Verification items for the finished model (mm, model axes). A direction names the side the tool comes from. Coordinates: 2 decimals unless noted, no trailing zeros. Loops run counter-clockwise (first coordinate to the right, second up) from the corner with the lowest first, then second, coordinate; pieces in that order, holes last. Notation, with made-up numbers: (72.5, 9.25) - (95.5, 9.25) arc R27 ccw to (95.5, 37.25) - close; hole circle Ø6 at (37, 7.25). An arc over 180 degrees is marked (long way). One line per item, written item: value. Start each with the question number.
(1) Section check D-D (z = 265). Record the boundary of the cut face in (x, y).
(2) Section check B-B (z = 12.7). Record the boundary of the cut face in (x, y) (1 decimal).
(3) Draft check along X on faces 1 (the face through (13, 1.587, 155)), 2 (the face through (25.4, 13, 155)), 3 (the face through (0, 13, 155)), 4 (the face through (0.805, 13.463, 198.237)). Enter one of: +X half, -X half, draft (parallel to the pull), parting line (faces both ways), or undercut.
(4) Set-up check for faces 5 (the face through (23.812, 13, 155)), 6 (the face through (0.8, 12.8, 279.4)): record each of +Z, -Z, +X, -X, +Y, -Y from which the full face is reachable in a straight line by a thin tool's end or side.
(5) Section check C-C (x = 10). Record the boundary of the cut face in (y, z).
(6) Section check A-A (z = 88.9). Record the boundary of the cut face in (x, y).
(7) Thickness scan on probe 1 along X at (y, z) = (6.5, 231.5); probe 2 along Y at (x, z) = (1.05, 114.3). Record the ranges inside material, lowest first. Write a range as [from, to].
```python
from build123d import *

# Parameters (mm, degrees)
SKETCH1_W           = 25.4
SKETCH1_H           = 25.4
SKETCH1_W_2         = 22.225
SKETCH1_H_2         = 22.225
BOSS_EXTRUDE1_DEPTH = 314.96
SKETCH3_R           = 2.54
CUT_EXTRUDE2_DEPTH  = 318.00176908
SKETCH4_R           = 2.54
CUT_EXTRUDE3_DEPTH  = 318.00176908


with BuildPart() as part:
    # Sketch1 → Boss-Extrude1 (new body)
    with BuildSketch(Plane.XY):
        with Locations((12.7, 12.7)):
            Rectangle(SKETCH1_W, SKETCH1_H)
        with Locations((12.7, 12.7)):
            Rectangle(SKETCH1_W_2, SKETCH1_H_2, mode=Mode.SUBTRACT)
    extrude(amount=BOSS_EXTRUDE1_DEPTH)

    # Sketch3 → Cut-Extrude2 (cut, through all)
    with BuildSketch(Plane(origin=(0, 25.4, 0), x_dir=(1, 0, 0), z_dir=(0, 1, 0))):
        with Locations(Location((15.875, -302.26, 0), (0, 0, 270))):
            Circle(SKETCH3_R)
        with Locations(Location((15.875, -12.7, 0), (0, 0, 270))):
            Circle(SKETCH3_R)
    extrude(amount=-CUT_EXTRUDE2_DEPTH, mode=Mode.SUBTRACT)

    # Sketch4 → Cut-Extrude3 (cut, through all)
    with BuildSketch(Plane(origin=(25.4, 0, 0), x_dir=(0, 0, -1), z_dir=(1, 0, 0))):
        with Locations((-302.26, 12.7)):
            Circle(SKETCH4_R)
        with Locations((-276.86, 12.7)):
            Circle(SKETCH4_R)
        with Locations((-251.46, 12.7)):
            Circle(SKETCH4_R)
        with Locations((-226.06, 12.7)):
            Circle(SKETCH4_R)
        with Locations((-200.66, 12.7)):
            Circle(SKETCH4_R)
        with Locations(Location((-114.3, 12.7, 0), (0, 0, 180))):
            Circle(SKETCH4_R)
        with Locations(Location((-88.9, 12.7, 0), (0, 0, 180))):
            Circle(SKETCH4_R)
        with Locations(Location((-63.5, 12.7, 0), (0, 0, 180))):
            Circle(SKETCH4_R)
        with Locations(Location((-38.1, 12.7, 0), (0, 0, 180))):
            Circle(SKETCH4_R)
        with Locations(Location((-12.7, 12.7, 0), (0, 0, 180))):
            Circle(SKETCH4_R)
    extrude(amount=-CUT_EXTRUDE3_DEPTH, mode=Mode.SUBTRACT)


solid = part.part
```
Responses:
1. outline: (0, 0) - (25.4, 0) - (25.4, 25.4) - (0, 25.4) - close; hole (1.59, 1.59) - (23.81, 1.59) - (23.81, 23.81) - (1.59, 23.81) - close
2. outline: (0, 0) - (13.3, 0) - (13.3, 1.6) - (1.6, 1.6) - (1.6, 10.2) - (0, 10.2) - close; (0, 15.2) - (1.6, 15.2) - (1.6, 23.8) - (13.3, 23.8) - (13.3, 25.4) - (0, 25.4) - close; (18.4, 0) - (25.4, 0) - (25.4, 10.2) - (23.8, 10.2) - (23.8, 1.6) - (18.4, 1.6) - close; (18.4, 23.8) - (23.8, 23.8) - (23.8, 15.2) - (25.4, 15.2) - (25.4, 25.4) - (18.4, 25.4) - close
3. face 1: undercut
3. face 2: +X half
3. face 3: -X half
3. face 4: draft
4. face 5: +Z, -Z
4. face 6: +X, -X
5. outline: (0, 0) - (1.59, 0) - (1.59, 314.96) - (0, 314.96) - close; (23.81, 0) - (25.4, 0) - (25.4, 314.96) - (23.81, 314.96) - close
6. outline: (0, 0) - (25.4, 0) - (25.4, 10.16) - (23.81, 10.16) - (23.81, 1.59) - (1.59, 1.59) - (1.59, 10.16) - (0, 10.16) - close; (0, 15.24) - (1.59, 15.24) - (1.59, 23.81) - (23.81, 23.81) - (23.81, 15.24) - (25.4, 15.24) - (25.4, 25.4) - (0, 25.4) - close
7. probe 1: x = [0, 1.59], [23.81, 25.4]
7. probe 2: y = [0, 10.16], [15.24, 25.4]
